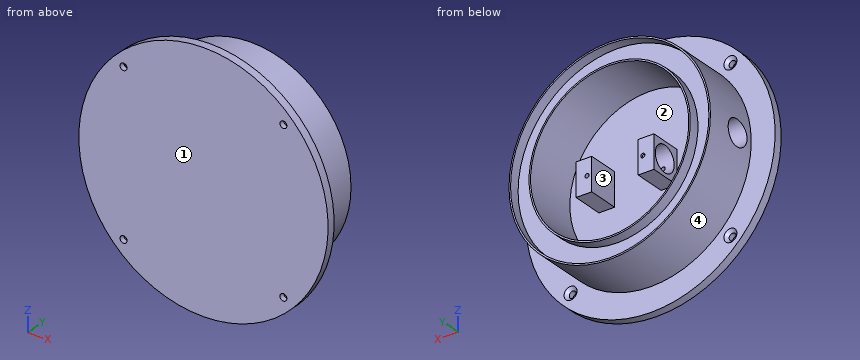
from build123d import *

# Parameters (mm, degrees)
SKETCH1_R                                           = 60.625
SKETCH1_R_2                                         = 45
BOSS_EXTRUDE1_DEPTH                                 = 4
SKETCH2_R                                           = 49
SKETCH2_R_2                                         = 45
BOSS_EXTRUDE2_DEPTH                                 = 27
SKETCH4_W                                           = 7.65
SKETCH4_H                                           = 16.2
BOSS_EXTRUDE4_DEPTH                                 = 8
BOSS_EXTRUDE4_2_DEPTH                               = 8
SKETCH5_R                                           = 45
BOSS_EXTRUDE5_DEPTH                                 = 5
SKETCH18_R                                          = 45.113728165
SKETCH18_R_2                                        = 38.5
BOSS_EXTRUDE6_DEPTH                                 = 31
CUT_EXTRUDE8_START                                  = -35
SKETCH11_R                                          = 6.25
CUT_EXTRUDE8_DEPTH                                  = 95.050498837
CSK_FOR_M3_COUNTERSUNK_FLAT_HEAD_SCREW1_D           = 3.4
CSK_FOR_M3_COUNTERSUNK_FLAT_HEAD_SCREW1_CSINK_D     = 6.3
CSK_FOR_M3_COUNTERSUNK_FLAT_HEAD_SCREW1_CSINK_ANGLE = 90
SKETCH27_R                                          = 1
CUT_EXTRUDE11_DEPTH                                 = 16
SKETCH28_R                                          = 48.25
SKETCH28_R_2                                        = 39.25
CUT_EXTRUDE12_DEPTH                                 = 5


with BuildPart() as part:
    # Sketch1 → Boss-Extrude1 (new body)
    with BuildSketch(Plane(origin=(0, 0, 0), x_dir=(1, 0, 0), z_dir=(0, 1, 0))):
        with Locations(Location((0, 0, 0), (0, 0, 270))):
            Circle(SKETCH1_R)
        with Locations(Location((0, 0, 0), (0, 0, 270))):
            Circle(SKETCH1_R_2, mode=Mode.SUBTRACT)
    extrude(amount=BOSS_EXTRUDE1_DEPTH)

    # Sketch2 → Boss-Extrude2 (add)
    with BuildSketch(Plane(origin=(0, 4, 0), x_dir=(1, 0, 0), z_dir=(0, 1, 0))):
        with Locations(Location((0, 0, 0), (0, 0, 270))):
            Circle(SKETCH2_R)
        with Locations(Location((0, 0, 0), (0, 0, 270))):
            Circle(SKETCH2_R_2, mode=Mode.SUBTRACT)
    extrude(amount=BOSS_EXTRUDE2_DEPTH)



with BuildPart() as body_2:
    # Sketch4 → Boss-Extrude4 (new, symmetric)
    with BuildSketch(Plane.XY):
        with Locations((-9.725, 12.1)):
            Rectangle(SKETCH4_W, SKETCH4_H)
    extrude(amount=BOSS_EXTRUDE4_DEPTH, both=True)


with BuildPart() as body_3:
    # Sketch4 → Boss-Extrude4 2 (new, symmetric)
    with BuildSketch(Plane.XY):
        with Locations((20.525, 12.1)):
            Rectangle(SKETCH4_W, SKETCH4_H)
    extrude(amount=BOSS_EXTRUDE4_2_DEPTH, both=True)


with BuildPart() as part_1:
    add(part.part)

    add(body_2.part)  # Boss-Extrude5 merges body 2

    add(body_3.part)  # Boss-Extrude5 merges body 3
    # Sketch5 → Boss-Extrude5 (add)
    with BuildSketch(Plane.XZ):
        with Locations(Location((0, 0, 0), (0, 0, 270))):
            Circle(SKETCH5_R)
    extrude(amount=-BOSS_EXTRUDE5_DEPTH)

    # Sketch18 → Boss-Extrude6 (add)
    with BuildSketch(Plane(origin=(0, 31, 0), x_dir=(1, 0, 0), z_dir=(0, 1, 0))):
        Circle(SKETCH18_R)
        with Locations(Location((0, 0, 0), (0, 0, 270))):
            Circle(SKETCH18_R_2, mode=Mode.SUBTRACT)
    extrude(amount=-BOSS_EXTRUDE6_DEPTH)

    # Sketch11 → Cut-Extrude8 (cut, through all)
    with BuildSketch(Plane(origin=(49, 0, 0), x_dir=(0, 0, -1), z_dir=(1, 0, 0)).offset(CUT_EXTRUDE8_START)):
        with Locations((0, 13)):
            Circle(SKETCH11_R)
    extrude(amount=-CUT_EXTRUDE8_DEPTH, mode=Mode.SUBTRACT)

    # CSK for M3 Countersunk Flat Head Screw1 (through all)
    with Locations(Plane(origin=(0, 4, 0), x_dir=(1, 0, 0), z_dir=(0, 1, 0))):
        with Locations((-38.890872965, 38.890872965), (-38.890872965, -38.890872965), (38.890872965, -38.890872965), (38.890872965, 38.890872965)):
            CounterSinkHole(CSK_FOR_M3_COUNTERSUNK_FLAT_HEAD_SCREW1_D / 2, CSK_FOR_M3_COUNTERSUNK_FLAT_HEAD_SCREW1_CSINK_D / 2, counter_sink_angle=CSK_FOR_M3_COUNTERSUNK_FLAT_HEAD_SCREW1_CSINK_ANGLE)

    # Sketch27 → Cut-Extrude11 (cut)
    with BuildSketch(Plane(origin=(0, 20.2, 0), x_dir=(1, 0, 0), z_dir=(0, 1, 0))):
        with Locations(Location((-8.175, 0, 0), (0, 0, 270))):
            Circle(SKETCH27_R)
        with Locations(Location((18.975, 0, 0), (0, 0, 270))):
            Circle(SKETCH27_R)
    extrude(amount=-CUT_EXTRUDE11_DEPTH, mode=Mode.SUBTRACT)

    # Sketch28 → Cut-Extrude12 (cut)
    with BuildSketch(Plane(origin=(0, 31, 0), x_dir=(1, 0, 0), z_dir=(0, 1, 0))):
        with Locations(Location((0, 0, 0), (0, 0, 270))):
            Circle(SKETCH28_R)
        with Locations(Location((0, 0, 0), (0, 0, 270))):
            Circle(SKETCH28_R_2, mode=Mode.SUBTRACT)
    extrude(amount=-CUT_EXTRUDE12_DEPTH, mode=Mode.SUBTRACT)


solid = part_1.part
Design review of the part built by this model. Coordinates are the model's own, in mm. Face numbers are marked on the shaded views. Coordinates: 2 decimals unless noted, no trailing zeros. Order: outer loops, then holes, each group sorted by start corner. A loop starts at its lowest first (then second) coordinate and runs counter-clockwise, first axis right, second up. Notation, with made-up numbers: (83, 46.5) -> (116, 46.5) arc R31 ccw to (116, 74.5) -> close; hole circle Ø5 at (39.25, 12). An arc over 180 degrees is marked (long way). Use one line per item in the form item = value. Start each with the question number.
(1) The part is to be moulded in two halves that separate along X. For the marked faces 1, 2, 3 and 4, say which applies: +X half, -X half, draft (parallel to the pull), parting line (faces both ways), or undercut.
(2) For probe 1 along X at (y, z) = (27.4, 0); probe 2 along X at (y, z) = (28.5, -9); probe 3 along Y at (x, z) = (-9.75, 0), list the stretches that pass through material, from the lowest coordinate up.
(3) Insertion check: pin 1 (14.5 mm diameter, centred on y = 13, z = 0, fed in from -X); pin 2 (10 mm diameter, centred on x = -39, z = 41, fed in from -Y); pin 3 (10 mm diameter, centred on x = 10.5, y = 8, fed in from +Z); pin 4 (2.5 mm diameter, centred on x = 21, y = 13, fed in from +Z). Each pin has a flat end and moves straight along its axis. Give the tip position at first contact, or say it passes through.
(4) Add section D-D on y = 24.5. State the section outline as (x, z) points, plus the area to 3 significant figures.
(5) Add section A-A on x = 0. State the section outline as (y, z) points (3 decimals).
(6) Add section C-C on z = 28. State the section outline as (x, y) points, plus the area to 3 significant figures.
(7) Add section B-B on y = 13. State the section outline as (x, z) points (3 decimals), plus the area to 3 significant figures.
Answer block:
q1.face_1 = draft
q1.face_2 = undercut
q1.face_3 = undercut
q1.face_4 = parting line
q2.probe_1 = -49 to -48.25, -39.25 to -38.5, 38.5 to 39.25, 48.25 to 49
q2.probe_2 = -48.17 to -47.4, -38.2 to -37.43, 37.43 to 38.2, 47.4 to 48.17
q2.probe_3 = 0 to 6.75, 19.25 to 20.2
q3.pin_1 = -49
q3.pin_2 = 0
q3.pin_3 = 60.16
q3.pin_4 = 44.84
q4.outline = circle Ø98 at (0, 0); hole circle Ø77 at (0, 0)
q4.area = 2,890 mm²
q5.outline = (0, -60.625) -> (4, -60.625) -> (4, -49) -> (31, -49) -> (31, -48.25) -> (26, -48.25) -> (26, -39.25) -> (31, -39.25) -> (31, -38.5) -> (5, -38.5) -> (5, 38.5) -> (31, 38.5) -> (31, 39.25) -> (26, 39.25) -> (26, 48.25) -> (31, 48.25) -> (31, 49) -> (4, 49) -> (4, 60.625) -> (0, 60.625) -> close
q6.outline = (-53.77, 0) -> (53.77, 0) -> (53.77, 4) -> (40.21, 4) -> (40.21, 31) -> (39.29, 31) -> (39.29, 26) -> (27.51, 26) -> (27.51, 31) -> (26.42, 31) -> (26.42, 5) -> (-26.42, 5) -> (-26.42, 31) -> (-27.51, 31) -> (-27.51, 26) -> (-39.29, 26) -> (-39.29, 31) -> (-40.21, 31) -> (-40.21, 4) -> (-53.77, 4) -> close
q6.area = 1,110 mm²
q7.outline = (-48.6, -6.25) arc R49 ccw (long way) to (-48.6, 6.25) -> (-37.989, 6.25) arc R38.5 cw (long way) to (-37.989, -6.25) -> close; (-13.55, -8) -> (-5.9, -8) -> (-5.9, -6.25) -> (-13.55, -6.25) -> close; (-13.55, 6.25) -> (-5.9, 6.25) -> (-5.9, 8) -> (-13.55, 8) -> close; (16.7, -8) -> (24.35, -8) -> (24.35, 8) -> (16.7, 8) -> close; hole circle Ø2 at (18.975, 0)
q7.area = 2,900 mm²
